Can you work these out from the model? Positions are in its coordinate system, mm. A direction names the side the tool comes from. Coordinates: 2 decimals unless noted, no trailing zeros. Order: outer loops, then holes, each group sorted by start corner. A loop starts at its lowest first (then second) coordinate and runs counter-clockwise, first axis right, second up. Notation, with made-up numbers: M -5,69 L 2,69 A36 ccw 2,103 Z; hole C -35.75,20 d2. An arc over 180 degrees is marked long. Answer as a JSON object with one key per item and string values.
from build123d import *

# Parameters (mm, degrees)
BOSS_EXTRUDE1_DEPTH = 5
FILLET1_R           = 20


with BuildPart() as part:
    # Sketch1 → Boss-Extrude1 (new body)
    with BuildSketch(Plane.XY):
        with BuildLine():
            Line((13.25, -3), (16.25, -3))
            Line((16.25, -3), (16.25, -5))
            Line((16.25, -5), (17.5, -5))
            Line((17.5, -5), (17.5, -7))
            Line((17.5, -7), (16.25, -7))
            Line((16.25, -7), (16.25, -9))
            Line((16.25, -9), (22.5, -9))
            Line((22.5, -9), (22.5, 9))
            Line((22.5, 9), (-22.5, 9))
            Line((-22.5, 9), (-22.5, -9))
            Line((-22.5, -9), (-16.25, -9))
            Line((-16.25, -9), (-16.25, -7))
            Line((-16.25, -7), (-17.5, -7))
            Line((-17.5, -7), (-17.5, -5))
            Line((-17.5, -5), (-16.25, -5))
            Line((-16.25, -5), (-16.25, -3))
            Line((-16.25, -3), (-13.25, -3))
            Line((-13.25, -3), (-13.25, -5))
            Line((-13.25, -5), (-12, -5))
            Line((-12, -5), (-12, -7))
            Line((-12, -7), (-13.25, -7))
            Line((-13.25, -7), (-13.25, -9))
            Line((-13.25, -9), (-9.5, -9))
            ThreePointArc((-9.5, -9), (0, 0.5), (9.5, -9))
            Line((9.5, -9), (13.25, -9))
            Line((13.25, -9), (13.25, -7))
            Line((13.25, -7), (12, -7))
            Line((12, -7), (12, -5))
            Line((12, -5), (13.25, -5))
            Line((13.25, -5), (13.25, -3))
        make_face()
    extrude(amount=BOSS_EXTRUDE1_DEPTH)

    # Fillet1
    # the kernel refuses this fillet: 20 mm, written as the material it takes off along each edge
    with BuildSketch(Plane(origin=(22.5, 9, -49.749371855), x_dir=(0, -1, 0), z_dir=(0, 0, 1))) as fillet1_piece_1:
        with BuildLine():
            CenterArc((20, -19.899748742), FILLET1_R, 95.739170477, 84.260829523)
            Line((0, -19.899748742), (-0.4, -19.899748742))
            Line((-0.4, -19.899748742), (-0.4, 0))
            Line((-0.4, 0), (0, 0.4))
            ThreePointArc((0, 0.4), (9, 0.4), (17.96, 0.397994975))
            Line((17.96, 0.397994975), (18, 0))
        make_face()
    extrude(amount=104.498743711, mode=Mode.SUBTRACT)
    with BuildSketch(Plane(origin=(-22.5, 9, -49.749371855), x_dir=(1, 0, 0), z_dir=(0, 0, 1))) as fillet1_piece_2:
        with BuildLine():
            CenterArc((19.899748742, -20), FILLET1_R, 90, 84.260829523)
            Line((0, -18), (-0.397994975, -17.96))
            ThreePointArc((-0.397994975, -17.96), (-0.4, -9), (-0.4, 0))
            Line((-0.4, 0), (0, 0.4))
            Line((0, 0.4), (19.899748742, 0.4))
            Line((19.899748742, 0.4), (19.899748742, 0))
        make_face()
    extrude(amount=104.498743711, mode=Mode.SUBTRACT)


solid = part.part
Item 1: I want a section at A-A, the plane y = -6. Write out the boundary of the cut face in (x, z), plus the area to 3 significant figures.
Answers follow:
{"outline": "M -21.97,0 L -17.5,0 L -17.5,5 L -21.97,5 Z; M -12,0 L -9.01,0 L -9.01,5 L -12,5 Z; M 9.01,0 L 12,0 L 12,5 L 9.01,5 Z; M 17.5,0 L 21.97,0 L 21.97,5 L 17.5,5 Z", "area": "74.5 mm^2"}
Item 2: I want a section at C-C, the plane y = -2.25. Write out the boundary of the cut face in (x, z).
Answers follow:
{"outline": "M -20.58,0 L -6.68,0 L -6.68,5 L -20.58,5 Z; M 6.68,0 L 20.58,0 L 20.58,5 L 6.68,5 Z"}
Item 3: I want a section at D-D, the plane x = 0. Write out the boundary of the cut face in (y, z).
Answers follow:
{"outline": "M 0.5,0 L 9,0 L 9,5 L 0.5,5 Z"}
Item 4: If we mould it in two halves opening along X, with no side actions, what happens to faces 4 (the flat face through (-15, -3, 2)), 5 (the flat face through (-11, -9, 2)), 6 (the cylindrical face through (-15.86, 3.97, 2.46))? For each: pulls with the +X half, pulls with the -X half, needs draft (parallel to the pull), parting line crosses it, or undercut.
Answers follow:
{"face 4": "undercut", "face 5": "needs draft", "face 6": "pulls with the -X half"}
Item 5: I'm going to push flat-ended pins straight in: pin 1 (2 mm diameter, centred on y = -6, z = 4, fed in from +X); pin 2 (3 mm diameter, centred on y = 6.5, z = 4, fed in from -X); pin 3 (2 mm diameter, centred on y = -4, z = 1.5, fed in from -X). Where does each tip first touch, or does it pass through?
Answers follow:
{"pin 1": "stops at x = 22.2", "pin 2": "stops at x = -14.6", "pin 3": "stops at x = -21.68"}
Item 6: Please list where these lines run through material, in increasing order: line 1 (X direction, y = -4, z = 4.25); line 2 (X direction, y = -6.5, z = 0.9); line 3 (Y direction, x = 12.5, z = 3.65).
Answers follow:
{"line 1": "x = -21.34 to -16.25, -13.25 to -8.08, 8.08 to 13.25, 16.25 to 21.34", "line 2": "x = -22.09 to -17.5, -12 to -9.17, 9.17 to 12, 17.5 to 22.09", "line 3": "y = -9 to -7, -5 to 6.38"}
Item 7: Which directions (+Z, -Z, +X, -X, +Y, -Y) give clear straight access to the entire face, cutting with the end or side of a thin tool? Please do faces 1 (the flat face through (-16.25, -8, 2)), 2 (the flat face through (11, -9, 2)), 3 (the flat face through (12, -6, 2)).
Answers follow:
{"face 1": "+Z, -Z, -Y", "face 2": "+Z, -Z, +X, -X, -Y", "face 3": "+Z, -Z"}
